Verification items for the finished model (mm, model axes). Face numbers are marked on the shaded views. A direction names the side the tool comes from. Coordinates: 2 decimals unless noted, no trailing zeros. Loops run counter-clockwise (first coordinate to the right, second up) from the corner with the lowest first, then second, coordinate; pieces in that order, holes last. Notation, with made-up numbers: (83, 80) - (94, 80) arc R9 ccw to (94, 91) - close; hole circle Ø7 at (-22.5, 80.25). An arc over 180 degrees is marked (long way). One line per item, written item: value. Start each with the question number.
(1) Section check A-A (z = 0). Record the boundary of the cut face in (x, y), plus the area to 3 significant figures.
(2) Section check B-B (y = -2.5). Record the boundary of the cut face in (x, z).
(3) Draft check along Z on the marked faces 1, 2 and 3. Enter one of: +Z half, -Z half, draft (parallel to the pull), parting line (faces both ways), or undercut.
(4) Set-up check for the marked faces 4, 5 and 6: record each of +Z, -Z, +X, -X, +Y, -Y from which the full face is reachable in a straight line by a thin tool's end or side.
(5) Gauge pin test, flat ends, axial feed: P1, Ø5, axis at y = 2, z = 4.5, coming from the -X side; P2, Ø2, axis at x = -2, z = 1.5, coming from the -Y side; P3, Ø2, axis at y = -1.5, z = -3, coming from the +X side. Record the tip position at first contact, or that the pin passes through.
(6) Section check C-C (y = 2). Record the boundary of the cut face in (x, z), plus the area to 3 significant figures.
(7) Thickness scan on probe 1 along Y at (x, z) = (-7, -5); probe 2 along X at (y, z) = (2.5, 0); probe 3 along X at (y, z) = (-1, 1.5). Record the ranges inside material, lowest first. Write a range as [from, to].
```python
from build123d import *

# Parameters (mm, degrees)
SKETCH_2_W          = 9.419019416
SKETCH_2_H          = 11.792672783
CUT_EXTRUDE_1_DEPTH = 1
FILLET_1_R          = 0.2
CHAMFER_1_SIZE      = 0.7
FILLET_2_R          = 0.2
FILLET_3_R          = 1
EXTRUDE_1_DEPTH     = 2


with BuildPart() as part:
    # 草图1 → 旋转1 (revolve)
    with BuildSketch(Plane.XY, mode=Mode.PRIVATE) as revolve_1_sk:
        Polygon((-1.596153846, 5), (-0.096153846, 5), (-0.096153846, 0), (4.403846154, 0), (4.403846154, -2), (-1.596153846, -2), align=None)
    revolve(revolve_1_sk.sketch.rotate(Axis((-3.596153846, 17.535042267, 0), (0, -1, 0)), 180), axis=Axis((-3.596153846, 17.535042267, 0), (0, -1, 0)))

    # 草图2 → 切除-拉伸1 (cut, symmetric)
    with BuildSketch(Plane.XY):
        with Locations((1.113355862, -0.208425672)):
            Rectangle(SKETCH_2_W, SKETCH_2_H)
    extrude(amount=CUT_EXTRUDE_1_DEPTH, both=True, mode=Mode.SUBTRACT)

    # 圆角1
    fillet_1_edges = [part.edges().sort_by_distance(p)[0] for p in [
        (-7.096153846, 5, 0),
    ]]
    fillet(fillet_1_edges, radius=FILLET_1_R)

    # 倒角1
    chamfer_1_edges = [part.edges().sort_by_distance(p)[0] for p in [
        (-11.596153846, 0, 0),
    ]]
    chamfer(chamfer_1_edges, length=CHAMFER_1_SIZE)

    # 圆角2
    fillet_2_edges = [part.edges().sort_by_distance(p)[0] for p in [
        (-11.596153846, -2, 0),
    ]]
    fillet(fillet_2_edges, radius=FILLET_2_R)

    # 圆角3
    fillet_3_edges = [part.edges().sort_by_distance(p)[0] for p in [
        (-7.096153846, 0, 0),
    ]]
    fillet(fillet_3_edges, radius=FILLET_3_R)

    # 草图3 → 凸台-拉伸1 (add)
    with BuildSketch(Plane.XZ.offset(2)):
        with BuildLine():
            Line((2.826462443, -1), (3.836880528, -1))
            ThreePointArc((3.836880528, -1), (-11.096153846, 0), (3.836880528, 1))
            Line((3.836880528, 1), (2.826462443, 1))
            ThreePointArc((2.826462443, 1), (-10.096153846, 0), (2.826462443, -1))
        make_face()
    extrude(amount=EXTRUDE_1_DEPTH)


solid = part.part
```
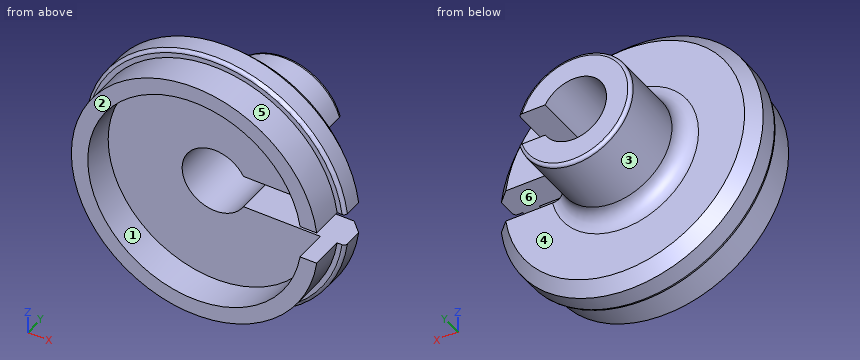
Responses:
1. outline: (-11.6, -1.8) arc R0.2 ccw to (-11.4, -2) - (-11.1, -2) - (-11.1, -4) - (-10.1, -4) - (-10.1, -2) - (-5.6, -2) - (-5.6, 5) - (-6.9, 5) arc R0.2 ccw to (-7.1, 4.8) - (-7.1, 1) arc R1 cw to (-8.1, 0) - (-10.9, 0) - (-11.6, -0.7) - close
1. area: 21.5 mm²
2. outline: (2.83, -1) arc R6.5 cw (long way) to (2.83, 1) - (3.84, 1) arc R7.5 ccw (long way) to (3.84, -1) - close
3. face 1: undercut
3. face 2: draft
3. face 3: parting line
4. face 4: +Y
4. face 5: -Y
4. face 6: +X, +Y, -Y
5. P1: stops at x = -10.33
5. P2: stops at y = -2
5. P3: stops at x = 4.15
6. outline: (-1.86, -1) arc R2 cw (long way) to (-1.86, 1) - (-0.24, 1) arc R3.5 ccw (long way) to (-0.24, -1) - close
6. area: 22.8 mm²
7. probe 1: y = [-2, 0]
7. probe 2: x = [-7.1, -5.6]
7. probe 3: x = [-11.45, -4.92], [-2.27, 4.26]
